Model file for the job. Use its own axes, mm. Face numbers are marked on the shaded views. A direction names the side the tool comes from. Coordinates: 2 decimals unless noted, no trailing zeros. Order: outer loops, then holes, each group sorted by start corner. A loop starts at its lowest first (then second) coordinate and runs counter-clockwise, first axis right, second up. Notation, with made-up numbers: M -10,-33.75 L -1,-33.75 A10 ccw -1,-23.75 Z; hole C 60.5,5 d8. An arc over 180 degrees is marked long. Return JSON: item names as keys, results as strings.
```python
from build123d import *

# Parameters (mm, degrees)
F1_DEPTH = 109
F0_W     = 3.5
F0_H     = 56.5
F2_DEPTH = 50
F3_R     = 20


with BuildPart() as f1:
    # F0 (on Right) → F1 (new body, symmetric)
    with BuildSketch(Plane.YZ):
        Polygon((-415.420956, -354.475219), (-415.420956, -357.975219), (-411.920956, -357.975219), (-235.420956, -357.975219), (-235.420956, -354.475219), align=None)
    extrude(amount=F1_DEPTH, both=True)

    # F0 (on Right) → F2 (join, symmetric)
    with BuildSketch(Plane.YZ):
        with Locations((-413.670956, -386.225219)):
            Rectangle(F0_W, F0_H)
        Polygon((-415.420956, -354.475219), (-415.420956, -357.975219), (-411.920956, -357.975219), (-235.420956, -357.975219), (-235.420956, -354.475219), align=None)
    extrude(amount=F2_DEPTH, both=True)

    # F3
    f3_edges = [f1.edges().sort_by_distance(p)[0] for p in [
        (109, -235.420956, -356.225219),
        (-109, -235.420956, -356.225219),
        (-109, -415.420956, -356.225219),
        (109, -415.420956, -356.225219),
    ]]
    fillet(f3_edges, radius=F3_R)


solid = f1.part
```
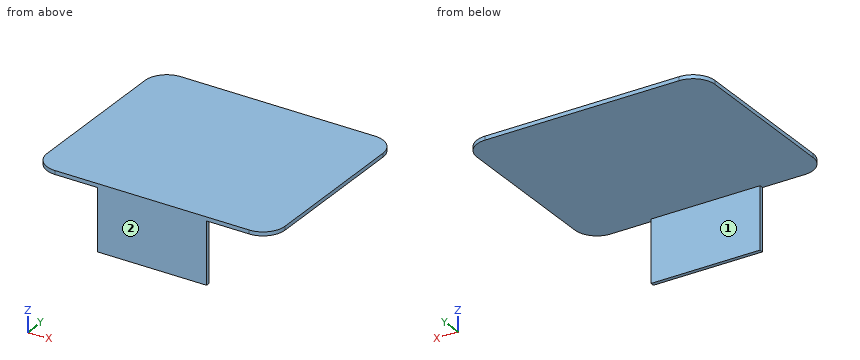
Item 1: Wall check: line 1 (Z direction, x = 74, y = -370.5); line 2 (Y direction, x = -24, z = -360). Give the ranges that are in metal, low to high.
Check result:
{"line 1": "z = -357.98 to -354.48", "line 2": "y = -415.42 to -411.92"}
Item 2: 3-axis set-ups, long thin cutter, end or side, ignore diameter. For the marked faces 1 and 2: which of +Z, -Z, +X, -X, +Y, -Y reach the whole face in a straight line?
Check result:
{"face 1": "-Z, +X, -X, +Y", "face 2": "+Z, -Z, +X, -X, -Y"}
Item 3: Saw through at B-B (z = -403). Write the cut outline in (x, y).
Check result:
{"outline": "M -50,-415.42 L 50,-415.42 L 50,-411.92 L -50,-411.92 Z"}
Item 4: Saw through at C-C (y = -366.5). Write the cut outline in (x, z), and give its area (3 significant figures).
Check result:
{"outline": "M -109,-357.98 L 109,-357.98 L 109,-354.48 L -109,-354.48 Z", "area": "763 mm2"}
Item 5: Drop flat-ended pins along their axis: pin 1 Ø17 at (x, z) = (3.5, -391) entering from +Y; pin 2 Ø4 at (y, z) = (-414.5, -397.5) entering from -X; pin 3 Ø1.5 at (x, y) = (-62.5, -267) entering from -Z. Give the stop position or say it passes through.
Check result:
{"pin 1": "stops at y = -411.92", "pin 2": "stops at x = -50", "pin 3": "stops at z = -357.98"}
Item 6: Saw through at A-A (x = -26). Write the cut outline in (y, z).
Check result:
{"outline": "M -415.42,-414.48 L -411.92,-414.48 L -411.92,-357.98 L -235.42,-357.98 L -235.42,-354.48 L -415.42,-354.48 Z"}
